Answer from the drawing. Dimensions are ordinates in mm from the lowest x, y and z of the part. Coordinates: 2 decimals unless noted, no trailing zeros. Write each loop counter-clockwise with the first axis right and the second up, starting at its lowest first coordinate (ties: lowest second). Pieces come first, ordered by that corner, then holes.
(1) The part is cut by section A-A, the plane y = 4.75. Determine the outline of the cut face in (x, z).
(2) Straight lines are drawn through the part: line 1 along X through (y, z) = (7.75, 1); line 2 along X through (y, z) = (11.75, 0.9); line 3 along Y through (x, z) = (105.5, 0.55). For each, find the intervals that lie inside material, in ascending order.
(3) The part is cut by section B-B, the plane z = 0.6. Determine the outline of the cut face in (x, y).
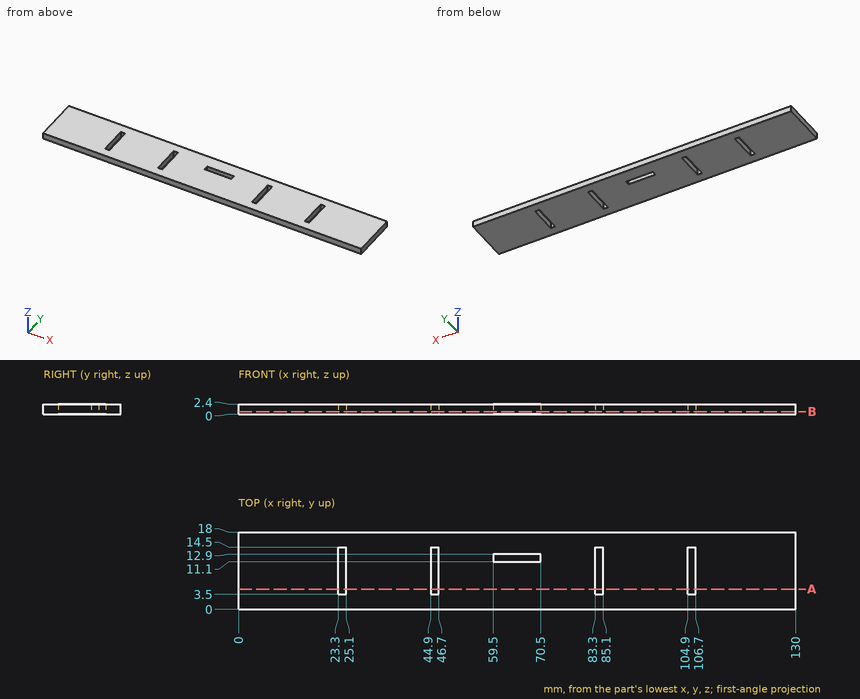
Computed:
1. outline: (0, 0) - (23.3, 0) - (23.3, 2.4) - (0, 2.4) - close; (25.1, 0) - (44.9, 0) - (44.9, 2.4) - (25.1, 2.4) - close; (46.7, 0) - (83.3, 0) - (83.3, 2.4) - (46.7, 2.4) - close; (85.1, 0) - (104.9, 0) - (104.9, 2.4) - (85.1, 2.4) - close; (106.7, 0) - (130, 0) - (130, 2.4) - (106.7, 2.4) - close
2. line 1: x = 0 to 23.3, 25.1 to 44.9, 46.7 to 83.3, 85.1 to 104.9, 106.7 to 130
2. line 2: x = 0 to 23.3, 25.1 to 44.9, 46.7 to 59.5, 70.5 to 83.3, 85.1 to 104.9, 106.7 to 130
2. line 3: y = 0 to 3.5, 14.5 to 18
3. outline: (0, 0) - (130, 0) - (130, 18) - (0, 18) - close; hole (23.3, 3.5) - (25.1, 3.5) - (25.1, 14.5) - (23.3, 14.5) - close; hole (44.9, 3.5) - (46.7, 3.5) - (46.7, 14.5) - (44.9, 14.5) - close; hole (59.5, 11.1) - (70.5, 11.1) - (70.5, 12.9) - (59.5, 12.9) - close; hole (83.3, 3.5) - (85.1, 3.5) - (85.1, 14.5) - (83.3, 14.5) - close; hole (104.9, 3.5) - (106.7, 3.5) - (106.7, 14.5) - (104.9, 14.5) - close
